Design review of the part shown in the three views and the two pictorial views. Dimensions are in mm from the part's minimum x, y and z. A direction names the side the tool comes from. Coordinates: 2 decimals unless noted, no trailing zeros. Order: outer loops, then holes, each group sorted by start corner. A loop starts at its lowest first (then second) coordinate and runs counter-clockwise, first axis right, second up. Notation, with made-up numbers: (-14.5, 83.5) -> (43.5, 83.5) arc R31 cw to (43.5, 108.5) -> close; hole circle Ø4 at (7.25, 85.5). An arc over 180 degrees is marked (long way). Answer as a JSON object with one key per item and string values. Group by question number.
1) Add section B-B, the plane x = 3.5. Write out the cut boundary in (y, z), then the cut area to 3 significant figures.
2) Wall thickness on L1, parallel to X at y = 2, z = 0.5; L2, parallel to X at y = 5, z = 1.25 (1 decimal); L3, parallel to Z at x = 11, y = 1.75: over which ranges is each line inside the solid? List them lowest first.
3) Add section C-C, the plane z = 6. Count the separate pieces of the cut face and the enclosed holes in it, then the cut area to 3 significant figures.
4) Add section A-A, the plane y = 3.5. Write out the cut boundary in (x, z) (1 decimal).
5) Draft analysis for pull direction Y (two halves, no side actions). For the marked faces 3, 4 and 5, state which applies: +Y half, -Y half, draft (parallel to the pull), parting line (faces both ways), or undercut.
6) Machinability: for the marked faces 1 and 2, which of the approach directions +Z, -Z, +X, -X, +Y, -Y give a long, thin tool a straight path to every point of the face, cutting with its end or side? Answer none if there is none.
7) For pin 1 (3 mm diameter, centred on x = 9.73, y = 3.18, fed in from -Z), flat-tipped, find the tip position at first contact; note if it passes through.
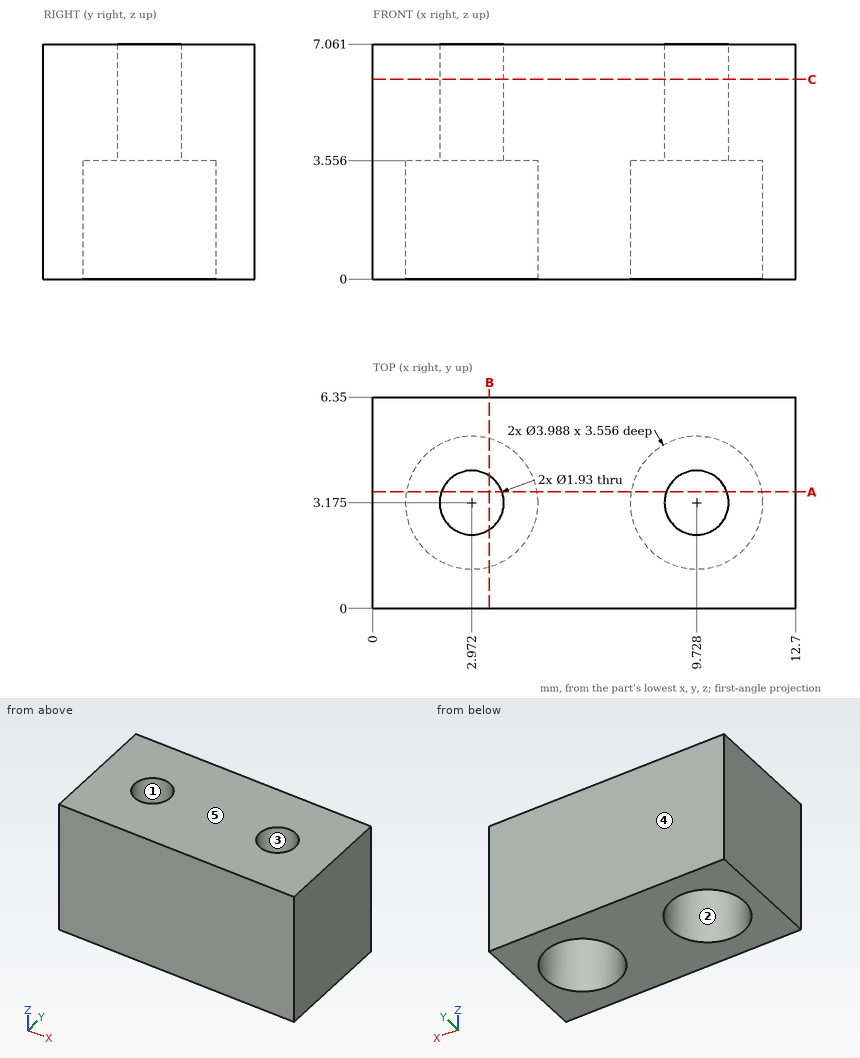
Output values:
{
 "1": {"outline": "(0, 0) -> (1.25, 0) -> (1.25, 3.56) -> (2.37, 3.56) -> (2.37, 7.06) -> (0, 7.06) -> close; (3.98, 3.56) -> (5.1, 3.56) -> (5.1, 0) -> (6.35, 0) -> (6.35, 7.06) -> (3.98, 7.06) -> close", "area": "25.5 mm²"},
 "2": {"L1": "x = 0 to 1.36, 4.58 to 8.12, 11.34 to 12.7", "L2": "x = 0 to 2.2, 3.8 to 8.9, 10.5 to 12.7", "L3": "z = 3.56 to 7.06"},
 "3": {"separate pieces": "1", "enclosed holes": "2", "area": "74.8 mm²"},
 "4": {"outline": "(0, 0) -> (1, 0) -> (1, 3.6) -> (2.1, 3.6) -> (2.1, 7.1) -> (0, 7.1) -> close; (3.9, 3.6) -> (4.9, 3.6) -> (4.9, 0) -> (7.8, 0) -> (7.8, 3.6) -> (8.8, 3.6) -> (8.8, 7.1) -> (3.9, 7.1) -> close; (10.6, 3.6) -> (11.7, 3.6) -> (11.7, 0) -> (12.7, 0) -> (12.7, 7.1) -> (10.6, 7.1) -> close"},
 "5": {"face 3": "undercut", "face 4": "+Y half", "face 5": "draft"},
 "6": {"face 1": "+Z, -Z", "face 2": "-Z"},
 "7": {"pin 1": "stops at z = 3.56"}
}
